Verification items for the finished model (mm, model axes). A direction names the side the tool comes from. Give positions to 0.01 mm unless a question says otherwise; leave off trailing zeros. Loops run counter-clockwise (first coordinate to the right, second up) from the corner with the lowest first, then second, coordinate; pieces in that order, holes last. Notation, with made-up numbers: (20.5, -20.75) -> (44.5, -20.75) arc R23 cw to (44.5, -2.75) -> close; hole circle Ø6 at (-38, -26). An arc over 180 degrees is marked (long way). Answer in a Markdown table with one row per item. Add a question column.
Q1. Gauge pin test, flat ends, axial feed: P1, Ø3, axis at x = -16.5, y = -2, coming from the -Z side; P2, Ø6, axis at x = -35, y = -17, coming from the +Z side; P3, Ø12, axis at y = -10.5, z = 40.5, coming from the -X side. Record the tip position at first contact, or that the pin passes through.
Q2. Section check A-A on x = 53. Enter the section's corners in (y, z).
Q3. Material ranges on probe 1 along Z at (x, y) = (-32.5, -1.5); probe 2 along X at (y, z) = (-26, 32.5); probe 3 along Z at (x, y) = (-27, -34), recorded low to high.
Q4. Set-up check for faces 1 (the face through (16.822, 2.275, 37.325)), 2 (the face through (-58.965, -12.718, 22.465)): record each of +Z, -Z, +X, -X, +Y, -Y from which the full face is reachable in a straight line by a thin tool's end or side.
Q5. Section check B-B on z = 34. Enter the section's corners in (x, y).
```python
from build123d import *

# Parameters (mm, degrees)
F0_W     = 150
F0_H     = 50
F1_DEPTH = 25
F3_DEPTH = 30
F4_R     = 5
F5_SIZE  = 5


with BuildPart() as f1:
    # F0 (on Top) → F1 (new body)
    with BuildSketch(Plane.XY):
        with Locations((13.5704912245, -12.3678184533)):
            Rectangle(F0_W, F0_H)
    extrude(amount=F1_DEPTH)

    # F2 (on face) → F3 (join)
    with BuildSketch(Plane.XY.offset(25)):
        with BuildLine():
            Line((-1.4295087755, -12.3678184533), (28.5704912245, -12.3678184533))
            ThreePointArc((28.5704912245, -12.3678184533), (13.5704912245, 2.6321815467), (-1.4295087755, -12.3678184533))
        make_face()
        with BuildLine():
            ThreePointArc((-1.4295087755, -12.3678184533), (13.5704912245, -27.3678184533), (28.5704912245, -12.3678184533))
            Line((28.5704912245, -12.3678184533), (-1.4295087755, -12.3678184533))
        make_face()
    extrude(amount=F3_DEPTH)

    # F4
    f4_edges = [f1.edges().sort_by_distance(p)[0] for p in [
        (28.570491, -12.367818, 55),
    ]]
    fillet(f4_edges, radius=F4_R)

    # F5
    f5_edges = [f1.edges().sort_by_distance(p)[0] for p in [
        (-61.429509, -12.367818, 25),
        (13.570491, -37.367818, 25),
        (13.570491, 12.632182, 25),
        (88.570491, -12.367818, 25),
    ]]
    chamfer(f5_edges, length=F5_SIZE)


solid = f1.part
```
Taken from the geometry:
| question | item | result |
|---|---|---|
| 1 | P1 | stops at z = 0 |
| 1 | P2 | stops at z = 25 |
| 1 | P3 | stops at x = -1.43 |
| 2 | outline | (-37.37, 0) -> (12.63, 0) -> (12.63, 20) -> (7.63, 25) -> (-32.37, 25) -> (-37.37, 20) -> close |
| 3 | probe 1 | z = 0 to 25 |
| 3 | probe 2 | x = 7.31 to 19.83 |
| 3 | probe 3 | z = 0 to 23.37 |
| 4 | face 1 | +Z |
| 4 | face 2 | +Z, -X, +Y, -Y |
| 5 | outline | circle Ø30 at (13.57, -12.37) |
